Answer from the drawing. Dimensions are ordinates in mm from the lowest x, y and z of the part. A direction names the side the tool comes from. Give positions to 0.01 mm unless a question says otherwise; leave off trailing zeros. Write each loop counter-clockwise with the first axis right and the second up, starting at its lowest first coordinate (ties: lowest second). Pieces come first, ordered by that corner, then holes. Notation, with made-up numbers: M 50.25,73 L 99.25,73 A17 ccw 99.25,101 Z; hole C 46.25,18 d5. An arc over 180 degrees is marked long. Put each result on its own line as item: value.
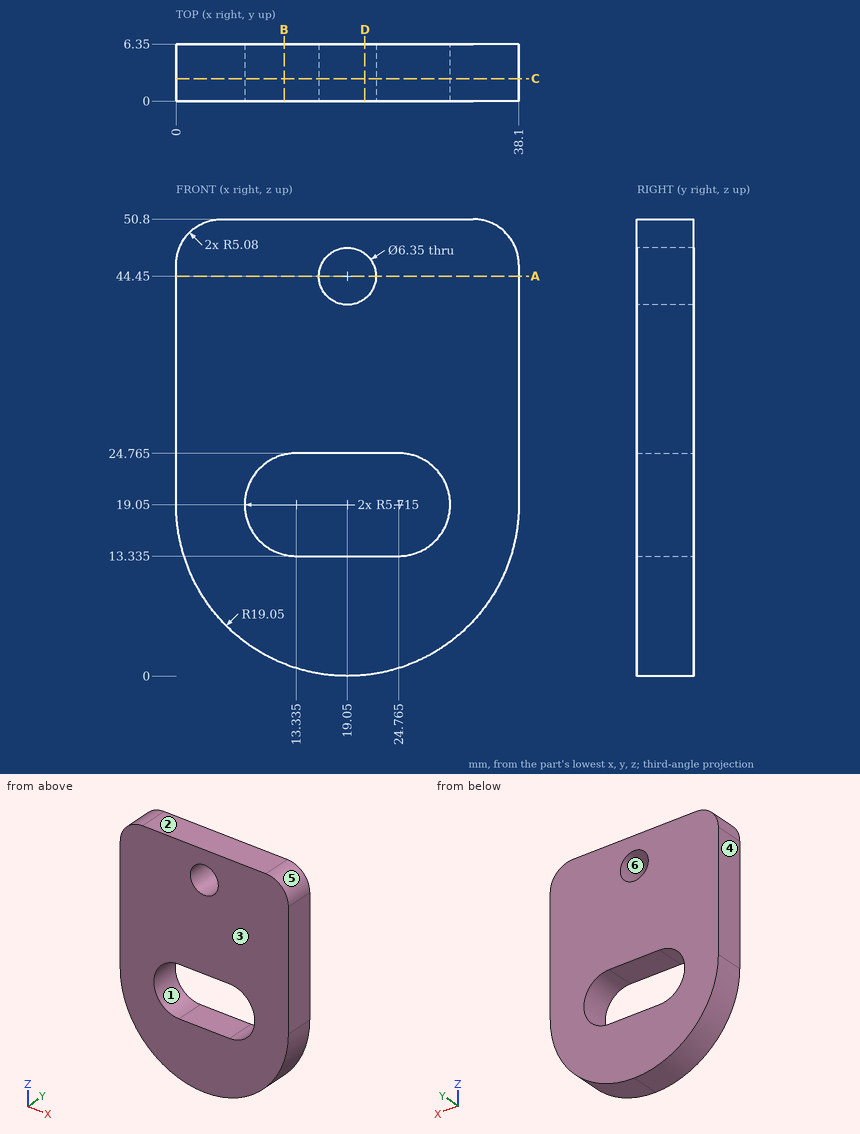
(1) Section B-B on x = 12 is taken. Determine the outline of the cut face in (y, z).
Result:
outline: M 0,1.35 L 6.35,1.35 L 6.35,13.49 L 0,13.49 Z; M 0,24.61 L 6.35,24.61 L 6.35,50.8 L 0,50.8 Z
(2) For a pull along X with two mould halves and no side action, classify the marked faces 3, 4, 5 and 6 as +X half, -X half, draft (parallel to the pull), parting line (faces both ways), or undercut.
Result:
face 3: draft
face 4: -X half
face 5: +X half
face 6: undercut
(3) Section A-A on z = 44.45 is taken. Determine the outline of the cut face in (x, y) (3 decimals), and give its area (3 significant figures).
Result:
outline: M 0,0 L 15.875,0 L 15.875,6.35 L 0,6.35 Z; M 22.225,0 L 38.1,0 L 38.1,6.35 L 22.225,6.35 Z
area: 202 mm²
(4) Section C-C on y = 2.5 is taken. Determine the outline of the cut face in (x, z) (3 decimals).
Result:
outline: M 0,19.05 A19.05 ccw 38.1,19.05 L 38.1,45.72 A5.08 ccw 33.02,50.8 L 5.08,50.8 A5.08 ccw 0,45.72 Z; hole M 13.335,13.335 L 24.765,13.335 A5.715 ccw 24.765,24.765 L 13.335,24.765 A5.715 ccw Z; hole C 19.05,44.45 d6.35
(5) Straight lines are drawn through the part: line 1 along Z through (x, y) = (20, 5) (3 decimals); line 2 along Z through (x, y) = (19, 4.25) (3 decimals); line 3 along X through (y, z) = (2.5, 44.45) (3 decimals). For each, find the intervals that lie inside material, in ascending order. Write a range as from..to.
Result:
line 1: z = 0.024..13.335, 24.765..41.42, 47.48..50.8
line 2: z = 0..13.335, 24.765..41.275, 47.625..50.8
line 3: x = 0..15.875, 22.225..38.1
(6) Which of the six approach directions +Z, -Z, +X, -X, +Y, -Y give full straight-line access (tool end or side, diameter ignored) to the marked faces 1 and 2?
Result:
face 1: +Y, -Y
face 2: +Z, +X, -X, +Y, -Y
(7) Given pin 1 Ø5.5 at (x, z) = (19.05, 44.45) entering from -Y; pin 2 Ø1 at (y, z) = (4, 5.5) entering from -X, each flat-ended and moving along its own axis, determine where each tip first touches the part or whether it passes through.
Result:
pin 1: passes through
pin 2: stops at x = 5.17
(8) Section D-D on x = 21 is taken. Determine the outline of the cut face in (y, z) (3 decimals), and give its area (3 significant figures).
Result:
outline: M 0,0.1 L 6.35,0.1 L 6.35,13.335 L 0,13.335 Z; M 0,24.765 L 6.35,24.765 L 6.35,41.944 L 0,41.944 Z; M 0,46.956 L 6.35,46.956 L 6.35,50.8 L 0,50.8 Z
area: 218 mm²
